from build123d import *

# Parameters (mm, degrees)
SKETCH_W     = 18
SKETCH_H     = 18
PAD_DEPTH    = 18
CHAMFER_SIZE = 16


with BuildPart() as part:
    # Sketch → Pad (new body)
    with BuildSketch(Plane.XY):
        with Locations((9, 9)):
            Rectangle(SKETCH_W, SKETCH_H)
    extrude(amount=PAD_DEPTH)

    # Chamfer
    chamfer_edges = [part.edges().sort_by_distance(p)[0] for p in [
        (9, 0, 18),
    ]]
    chamfer(chamfer_edges, length=CHAMFER_SIZE)


solid = part.part
Could you check a few things on this model? Use its own coordinates, in mm. Give positions to 0.01 mm unless a question says otherwise; leave off trailing zeros. Order: outer loops, then holes, each group sorted by start corner. A loop starts at its lowest first (then second) coordinate and runs counter-clockwise, first axis right, second up. Notation, with made-up numbers: (40.5, 17.5) -> (54.5, 17.5) arc R8 cw to (54.5, 25.5) -> close; hole circle Ø9 at (-33.75, 86.25). An arc over 180 degrees is marked (long way). Answer in a Markdown table with one row per item. Add a question column.
Item 1: Please list where these lines run through material, in increasing order: probe 1 along Y at (x, z) = (12.25, 5); probe 2 along Y at (x, z) = (14.25, 4.5); probe 3 along Z at (x, y) = (9.25, 11.5).
Item 2: Imagine slicing it at B-B (x = 3.25). List the corners of the cut face in (y, z) for me.
Item 3: Imagine slicing it at A-A (y = 10). List the corners of the cut face in (x, z) for me.
Item 4: I'm going to push flat-ended pins straight in: P1, Ø1, axis at x = 11.5, y = 12.5, coming from the +Z side; P2, Ø4, axis at x = 6, y = 6.5, coming from the +Z side; P3, Ø1, axis at x = 13, z = 10, coming from the -Y side. Where does each tip first touch, or does it pass through?
Item 5: Imagine slicing it at C-C (z = 8.5). List the corners of the cut face in (x, y) for me, and give its area (3 significant figures).
Result:
| question | item | result |
|---|---|---|
| 1 | probe 1 | 3 to 18 |
| 1 | probe 2 | 2.5 to 18 |
| 1 | probe 3 | 0 to 13.5 |
| 2 | outline | (0, 0) -> (18, 0) -> (18, 18) -> (16, 18) -> (0, 2) -> close |
| 3 | outline | (0, 0) -> (18, 0) -> (18, 12) -> (0, 12) -> close |
| 4 | P1 | z = 15 |
| 4 | P2 | z = 10.5 |
| 4 | P3 | y = 7.5 |
| 5 | outline | (0, 6.5) -> (18, 6.5) -> (18, 18) -> (0, 18) -> close |
| 5 | area | 207 mm2 |
